from build123d import *

# Parameters (mm, degrees)
F0_R     = 19.5456573821
F1_DEPTH = 112.014
F2_T     = -2.54


# Not quite as in the source:
# - a fillet or chamfer that OpenCascade refuses, or shapes differently, is made with other operations: its cross-section is extruded or revolved along the edge and cut away or added


with BuildPart() as f1:
    # F0 (on Front) → F1 (new body)
    with BuildSketch(Plane.XZ):
        Circle(F0_R)
    extrude(amount=F1_DEPTH)

    # F2
    f2_openings = [f1.faces().sort_by_distance(p)[0] for p in [
        (0, -112.014, 0),
    ]]
    offset(amount=F2_T, openings=f2_openings)

    # F3: chamfer of 5.08 on 1 edges, made by hand

    # F3_s1 → F3_t2 (revolve, cut)
    with BuildSketch(Plane.XY):
        Polygon((22.0856573821, -112.014), (17.0056573821, -106.934), (17.0056573821, -112.014), align=None)
    revolve(axis=Axis((0, -112.014, 0), (0, -1, 0)), mode=Mode.SUBTRACT)


solid = f1.part
Geometry check sheet. Reference: the model listing, model coordinates, mm. Give positions to 0.01 mm unless a question says otherwise; leave off trailing zeros. Order: outer loops, then holes, each group sorted by start corner. A loop starts at its lowest first (then second) coordinate and runs counter-clockwise, first axis right, second up. Notation, with made-up numbers: (50, 43.5) - (76, 43.5) arc R30 ccw to (76, 67.5) - close; hole circle Ø10 at (63.5, 22). An arc over 180 degrees is marked (long way). Answer as a JSON object with one key per item and string values.
(1) Cross-section at C-C (y = -48). Record the cut outline in (x, z).
Report:
{"outline": "circle Ø39.09 at (0, 0); hole circle Ø34.01 at (0, 0)"}
(2) Cross-section at B-B (z = 0). Record the cut outline in (x, y), then the cut area to 3 significant figures.
Report:
{"outline": "(-19.55, -109.47) - (-17.01, -106.93) - (-17.01, -2.54) - (17.01, -2.54) - (17.01, -106.93) - (19.55, -109.47) - (19.55, 0) - (-19.55, 0) - close", "area": "636 mm^2"}
(3) Cross-section at A-A (x = 0). Record the cut outline in (y, z).
Report:
{"outline": "(-109.47, -19.55) - (0, -19.55) - (0, 19.55) - (-109.47, 19.55) - (-106.93, 17.01) - (-2.54, 17.01) - (-2.54, -17.01) - (-106.93, -17.01) - close"}
(4) Draft check along Z on faces 1 (the conical face through (16.34, -107.06, 5.15)), 2 (the flat face through (0, -2.54, 0)), 3 (the cylindrical face through (-15.511, -53.971, -11.893)), 4 (the flat face through (0, 0, 0)). Enter one of: released by +Z, released by -Z, zero draft, split by the parting line, or undercut.
Report:
{"face 1": "undercut", "face 2": "undercut", "face 3": "split by the parting line", "face 4": "zero draft"}
(5) Material ranges on line 1 (X direction, y = -59, z = 0); line 2 (Y direction, x = -8.5, z = 7.5), recorded low to high.
Report:
{"line 1": "-19.55 to -17.01, 17.01 to 19.55", "line 2": "-2.54 to 0"}
(6) Depth check by flat-ended pin: pin 1 Ø10 at (x, z) = (4, 2) entering from -Y; pin 2 Ø2 at (y, z) = (-53, 11) entering from +X; pin 3 Ø5 at (y, z) = (-62.5, 8) entering from -X. Enter the tip coordinate at first touch or a pass-through.
Report:
{"pin 1": "y = -2.54", "pin 2": "x = 16.79", "pin 3": "x = -18.76"}
